Autodesk Inventor part; units mm, degrees
ref_plane "YZ Plane" through (0, 0, 0) normal (1, 0, 0) x (0, 1, 0)
ref_plane "XZ Plane" through (0, 0, 0) normal (0, 1, 0) x (-1, 0, 0)
ref_plane "XY Plane" through (0, 0, 0) normal (0, 0, 1) x (1, 0, 0)
sketch "Sketch2" plane through (0, 0, 0) normal (0, 0, 1) x (-1, 0, 0)
  circle A0 centre (0, 0) radius 25
  line L0 (0, 0) -> (20, 0) construction
  line L1 (0, 0) -> (20, 0) construction
  line L2 (0, 0) -> (20, 0) construction
  line L3 (0, 0) -> (20, 0) construction
  circle A1 centre (14.1421, 14.1421) radius 3.125
  circle A2 centre (-14.1421, 14.1421) radius 3.125
  circle A3 centre (-14.1421, -14.1421) radius 3.125
  circle A4 centre (14.1421, -14.1421) radius 3.125
  dimension "d0" = 50
  dimension "d10" = 6.25
  dimension "d11" = 6.25
  dimension "d12" = 6.25
  dimension "d13" = 6.25
extrude "Extrusion1" add sketch "Sketch2" along normal blind 3
sketch "Sketch19" plane through (0, 0, 3) normal (0, 0, 1) x (1, 0, 0)
  circle A0 centre (0, 0) radius 10
  dimension "d40" = 20
sketch "Sketch22" plane through (0, 0, 0) normal (0, 1, 0) x (-1, 0, 0)
  line L0 (25, 3) -> (-25, 3)
  line L1 (0, 3) -> (-8.6824, 52.2404)
  line L2 (0, 3) -> (50, 3) construction
  point P0 (0, 0)
  dimension "d41" = 50
  dimension "d42" = 100
sweep "Sweep4" add profiles "Sketch19" path "Sketch22" path curves L1
sketch "Sketch23" plane through (0, 0, 3) normal (0, 0, 1) x (1, 0, 0)
  circle A0 centre (0, 0) radius 8.5
  dimension "d45" = 17
sketch "Sketch25" plane through (0, 0, 0) normal (0, 1, 0) x (-1, 0, 0)
  line L0 (25, 3) -> (-25, 3)
  line L1 (0, 3) -> (-8.6824, 52.2404)
  line L2 (0, 3) -> (50, 3) construction
  point P0 (0, 0)
  dimension "d46" = 50
  dimension "d47" = 100
sweep "Sweep5" cut profiles "Sketch23" path "Sketch25" path curves L1
fillet "Fillet2" radius 3 1 edges at (-10, 0, 3)
properties part number "SoporteMarcador"
Input: part model. Units: mm. Frame: model coordinates. Give positions to 0.01 mm unless a question says otherwise; leave off trailing zeros. Loops run counter-clockwise (first coordinate to the right, second up) from the corner with the lowest first, then second, coordinate; pieces in that order, holes last.
1) Line query: L1, parallel to Z at x = 19, y = 3; L2, parallel to X at y = -2, z = 49; L3, parallel to X at y = 4, z = 44. Output: solid intervals per line, ascending.
A:
L1: z = 0 to 3
L2: x = -1.69 to -0.15, 16.37 to 17.91
L3: x = -1.94 to -0.27, 14.73 to 16.39
2) Section query D-D on x = 20.5. Return the cut outline in (y, z).
A:
outline: (-14.31, 0) - (14.31, 0) - (14.31, 3) - (-14.31, 3) - close
3) Section query A-A on x = -15.5. Return the cut outline in (y, z), and give its area (3 significant figures).
A:
outline: (-19.62, 0) - (-16.96, 0) - (-16.96, 3) - (-19.62, 3) - close; (-11.33, 0) - (11.33, 0) - (11.33, 3) - (-11.33, 3) - close; (16.96, 0) - (19.62, 0) - (19.62, 3) - (16.96, 3) - close
area: 83.9 mm2
4) Contact query for a flat-ended pin moving along its axis: pin 1 (8 mm diameter, centred on x = -14.14, y = -14.14, fed in from +Z). Output: stop coordinate, or through.
A:
pin 1: stops at z = 3
5) Mould query, pull axis Y, two halves, no side actions, for faces 1 (the cylindrical face through (14.82, 11.09, 1.48)), 2 (the flat face through (0, 0, 3)), 3 (the cylindrical face through (-23.846, 7.509, 1.479)), 4 (the flat face through (0, 0, 0)). Classes: released by +Y, released by -Y, zero draft, split by the parting line, or undercut.
A:
face 1: undercut
face 2: undercut
face 3: split by the parting line
face 4: zero draft
6) Section query B-B on y = -20. Return the cut outline in (x, z), and give its area (3 significant figures).
A:
outline: (-15, 0) - (15, 0) - (15, 3) - (-15, 3) - close
area: 90.0 mm2
7) Section query C-C on y = -12. Count the separate pieces of the cut face and the enclosed holes in it, and give its area (3 significant figures).
A:
separate pieces: 3
enclosed holes: 0
area: 105 mm2
